Check sheet for the modelled part. Datum: model origin and axes. Units: mm. A direction names the side the tool comes from. Give positions to 0.01 mm unless a question says otherwise; leave off trailing zeros. Write each loop counter-clockwise with the first axis right and the second up, starting at its lowest first coordinate (ties: lowest second). Pieces come first, ordered by that corner, then holes. Notation, with made-up numbers: (-15.5, 22.25) -> (40.5, 22.25) arc R25 ccw to (40.5, 57.25) -> close; hole circle Ø1 at (-33, -25). An arc over 180 degrees is marked (long way). Use a Markdown table: item, result. Add a question column.
1. Cross-section at A-A (z = 2). Enter the section's corners in (x, y), then the cut area to 3 significant figures.
2. Gauge pin test, flat ends, axial feed: P1, Ø1.5, axis at y = 7, z = 1, coming from the +X side; P2, Ø1.5, axis at x = 1, y = -2, coming from the +Z side; P3, Ø3, axis at x = -5.5, y = 4, coming from the -Z side. Record the tip position at first contact, or that the pin passes through.
3. Scan lines: probe 1 along Z at (x, y) = (-7.5, -4); probe 2 along Z at (x, y) = (1.5, -3); probe 3 along Y at (x, z) = (1.75, -3.5). Record each from-to range of solid material in increasing order. Write a range as [from, to].
4. Set-up check for faces 1 (the flat face through (0, 0, -4)), 2 (the cylindrical face through (0, -3, -4)), 3 (the cylindrical face through (-0.867, 3.905, -0.493)): record each of +Z, -Z, +X, -X, +Y, -Y from which the full face is reachable in a straight line by a thin tool's end or side.
5. Cross-section at B-B (z = -4.25). Enter the section's corners in (x, y), then the cut area to 3 significant figures.
from build123d import *

# Parameters (mm, degrees)
F0_W     = 4
F0_H     = 1
F2_SIZE  = 1
F3_R     = 1
F5_DEPTH = 5.5
F6_SIZE  = 0.3


with BuildPart() as f1:
    # F0 (on Front) → F1 (revolve)
    with BuildSketch(Plane.XZ):
        with BuildLine():
            ThreePointArc((9.5, 4), (4.8088460154, 2.877308569), (0, 2.5))
            Line((0, 2.5), (0, 0))
            Line((0, 0), (4, 0))
            Line((4, 0), (9.5, 0))
            Line((9.5, 0), (9.5, 4))
        make_face()
        with Locations((2, -0.5)):
            Rectangle(F0_W, F0_H)
    revolve(axis=Axis((0, 0, 1.25), (0, 0, -1)))

    # F2
    f2_edges = [f1.edges().sort_by_distance(p)[0] for p in [
        (-9.5, 0, 0),
    ]]
    chamfer(f2_edges, length=F2_SIZE)

    # F3
    f3_edges = [f1.edges().sort_by_distance(p)[0] for p in [
        (-9.5, 0, 4),
    ]]
    fillet(f3_edges, radius=F3_R)

    # F4 (on face) → F5 (join)
    with BuildSketch(Plane(origin=(0, 0, -1), x_dir=(1, 0, 0), z_dir=(0, 0, -1))):
        with BuildLine():
            Line((-3, 0), (3, 0))
            ThreePointArc((3, 0), (0, 3), (-3, 0))
        make_face()
    extrude(amount=F5_DEPTH)

    # F6
    f6_edges = [f1.edges().sort_by_distance(p)[0] for p in [
        (0, 0, -6.5),
        (0, -3, -6.5),
    ]]
    chamfer(f6_edges, length=F6_SIZE)


solid = f1.part
Worked answers:
| question | item | result |
|---|---|---|
| 1 | outline | circle Ø19 at (0, 0) |
| 1 | area | 284 mm² |
| 2 | P1 | stops at x = 7.15 |
| 2 | P2 | stops at z = 2.64 |
| 2 | P3 | stops at z = 0 |
| 3 | probe 1 | z = [0, 3.66] |
| 3 | probe 2 | z = [-1, 2.68] |
| 3 | probe 3 | y = [-2.44, 0] |
| 4 | face 1 | -Z, +X, -X, +Y |
| 4 | face 2 | -Z, -Y |
| 4 | face 3 | -Z |
| 5 | outline | (-3, 0) arc R3 ccw to (3, 0) -> close |
| 5 | area | 14.1 mm² |
